Geometry: final body of the model. Coordinates: model frame, mm. A direction names the side the tool comes from. Round coordinates to 2 decimals unless told otherwise and drop trailing zeros. Loops run counter-clockwise (first coordinate to the right, second up) from the corner with the lowest first, then second, coordinate; pieces in that order, holes last. Notation, with made-up numbers: (-22, 77.5) - (27, 77.5) arc R31 ccw to (27, 106.5) - close; hole circle Ø3 at (8.5, 26.5). An arc over 180 degrees is marked (long way). Use CSV: the item, a comma, the result in double quotes.
Autodesk Inventor part; units mm, degrees
ref_plane "РабПлоскость4" through (-4.5219, -7.4249, -3) normal (0, 0, 1) x (1, 0, 0)
ref_plane "РабПлоскость5" through (-4.5219, -7.4249, -3) normal (0, 0, 1) x (1, 0, 0)
ref_plane "YZ Plane" through (0, 0, 0) normal (1, 0, 0) x (0, 1, 0)
sketch "Эскиз1" plane through (0, 0, 0) normal (0, 0, 1) x (1, 0, 0)
  arc A0 (0.3914, -1.6228) -> (0.394, 1.6268) centre (2.903, 0) ccw construction
  circle A1 centre (2.903, 0) radius 2.9903
  circle A2 centre (2.903, 0) radius 6
  point P0 (0, 0)
  dimension "d0" = 12
extrude "Выдавливание1" add sketch "Эскиз1" along normal blind 24
ref_plane "РабПлоскость2" through (3.6207, 5.9569, 0) normal (-0.1196, -0.9928, 0) x (0.9928, -0.1196, 0)
ref_plane "РабПлоскость1" through (5.8216, 7.5048, 10) normal (-0.1196, -0.9928, 0) x (0.9928, -0.1196, 0)
sketch "Эскиз2" plane through (3.6207, 5.9569, 0) normal (-0.1196, -0.9928, 0) x (0.9928, -0.1196, 0)
  line L0 (6, 0) -> (-6, 0)
  line L1 (0, 0) -> (0, 19.3984) construction
  line L2 (0, 12.5) -> (0, 16.5) construction
  line L3 (2, 12.5) -> (2, 16.5)
  line L4 (-2, 16.5) -> (-2, 12.5)
  arc A0 (-2, 12.5) -> (2, 12.5) centre (0, 12.5) ccw
  arc A1 (2, 16.5) -> (-2, 16.5) centre (0, 16.5) ccw
  point P0 (-2.8822, 0)
  point P1 (0, 14.5)
  dimension "d0" = 12
  dimension "d3" = 4
  dimension "d4" = 4
  dimension "d5" = 14.5
extrude "Выдавливание2" cut sketch "Эскиз2" along normal blind 2.5
ref_plane "РабПлоскость3" through (2.903, 0, 19) normal (0, 0, -1) x (-1, 0, 0)
sketch "Эскиз3" plane through (2.903, 0, 19) normal (0, 0, -1) x (-1, 0, 0)
  point P0 (2.903, 0)
sketch "Эскиз4" plane through (2.903, 0, 19) normal (0, 0, -1) x (-1, 0, 0)
  circle A0 centre (0, 0) radius 6.5
  point P0 (2.903, 0)
  dimension "d12" = 13
extrude "Выдавливание3" add sketch "Эскиз4" against normal blind 20
sketch "Эскиз5" plane through (2.903, 0, 39) normal (0, 0, 1) x (1, 0, 0)
  circle A0 centre (0, 0) radius 5
  circle A1 centre (0, 0) radius 7.2744
  point P0 (-2.903, 0)
  dimension "d15" = 10
extrude "Выдавливание4" cut sketch "Эскиз5" against normal blind 19
sketch "Эскиз6" plane through (2.903, 0, 0) normal (0, 0, -1) x (-1, 0, 0)
  circle A0 centre (0, 0) radius 3
  circle A1 centre (0, 0) radius 5
  point P0 (2.903, 0)
  dimension "d18" = 6
  dimension "d19" = 10
ref_plane "РабПлоскость4" through (-4.5219, -7.4249, -3) normal (0, 0, 1) x (1, 0, 0)
sketch "Эскиз8" plane through (2.903, 0, 0) normal (0, 0, -1) x (-1, 0, 0)
  circle A0 centre (0, 0) radius 6
  point P0 (2.903, 0)
extrude "Выдавливание6" cut sketch "Эскиз8" against normal blind 9
sketch "Эскиз9" plane through (2.903, 0, 9) normal (0, 0, -1) x (-1, 0, 0)
  circle A0 centre (0, 0) radius 3
  circle A1 centre (0, 0) radius 5
  point P0 (2.903, 0)
  dimension "d24" = 6
  dimension "d25" = 10
ref_plane "РабПлоскость5" through (-4.5219, -7.4249, -3) normal (0, 0, 1) x (1, 0, 0)
extrude "Выдавливание7" add sketch "Эскиз9" along normal up to surface (12 mm away)
sketch "Эскиз10" plane through (2.903, 0, 39) normal (0, 0, 1) x (1, 0, 0)
  circle A0 centre (0, 0) radius 5
  point P0 (-2.903, 0)
extrude "Выдавливание8" add sketch "Эскиз10" along normal blind 62
sketch "Эскиз11" plane through (2.903, 0, 101) normal (0, 0, 1) x (1, 0, 0)
  line L0 (3.5, 4.5942) -> (9.6944, 4.5942)
  line L1 (9.6944, 4.5942) -> (9.6944, -5.4033)
  line L2 (9.6944, -5.4033) -> (3.5, -5.4033)
  line L3 (3.5, -5.4033) -> (3.5, 4.5942)
  circle A0 centre (0, 0) radius 5
  point P0 (-2.903, 0)
  point P1 (3.5, 3.5707)
  point P2 (3.5, -3.5707)
  dimension "d30" = 3.5
extrude "Выдавливание9" cut sketch "Эскиз11" against normal blind 30 contours A0 L3 picked at (3.7121, 0.9363)
sketch "Эскиз12" plane through (2.903, 0, 20) normal (0, 0, 1) x (1, 0, 0)
  circle A0 centre (0, 0) radius 5.5
  point P0 (-2.903, 0)
  dimension "d33" = 11
extrude "Выдавливание10" add sketch "Эскиз12" along normal blind 38.8
sketch "Эскиз13" plane through (6.403, -3.5707, 101) normal (1, 0, 0) x (0, 0, -1)
  point P0 (101, 3.5707)
sketch "Эскиз14" plane through (6.403, -3.5707, 101) normal (1, 0, 0) x (0, 0, -1)
  point P0 (101, 3.5707)
sketch "Эскиз15" plane through (6.403, -3.5707, 101) normal (1, 0, 0) x (0, 0, -1)
  line L0 (30, 0) -> (30, 7.1414)
  line L1 (30, 3.5707) -> (0, 3.5707) construction
  line L2 (0, 8.5707) -> (0, -1.4293)
  point P0 (101, 3.5707)
  point P1 (0, 7.1414)
  point P2 (0, 0)
  point P3 (7, 3.5707)
  point P4 (23, 3.5707)
  dimension "d36" = 7
  dimension "d37" = 7
hole "Отверстие1" at (6.403, 0, 94) at (6.403, 0, 78) direction (-1, 0, 0) diameter 3.242 depth 11.8 tip angle 118
sketch "Эскиз16" plane through (2.903, 0, 9) normal (0, 0, -1) x (-1, 0, 0)
  circle A0 centre (0, 0) radius 6
  point P0 (2.903, 0)
extrude "Выдавливание11" add sketch "Эскиз16" along normal blind 1
ref_plane "РабПлоскость6" through (2.903, 0, 10) normal (0, 0, -1) x (0.9928, -0.1196, 0)
sketch "Эскиз17" plane through (2.903, 0, 10) normal (0, 0, -1) x (0.9928, -0.1196, 0)
  circle A0 centre (0, 0) radius 5.65
  circle A1 centre (0, 0) radius 7.5447
  point P0 (-2.8822, 0.3472)
  dimension "d47" = 11.3
extrude "Выдавливание12" cut sketch "Эскиз17" along normal blind 1.2
sketch "Эскиз18" plane through (0, 0, 0) normal (0, 1, 0) x (-1, 0, 0)
  line L0 (-7.903, -3) -> (2.097, -3) construction
  line L1 (2.097, -3) -> (-7.903, -3)
  line L2 (-2.903, -3) -> (-2.903, 1.2) construction
  point P0 (0, 0)
  dimension "d50" = 4.2
hole "Отверстие2" at (2.903, 0, 1.2) direction (0, 1, 0) diameter 2.459 depth 8.8 tip angle 118
properties part number "Вал вертикальной оси"
Item 1: Pin query (flat end, axial travel): P1, Ø6, axis at x = 4.5, y = 1, coming from the -Z side; P2, Ø5, axis at x = -0.5, z = 29.5, coming from the +Y side; P3, Ø2, axis at y = -5, z = 74.5, coming from the -X side; P4, Ø2, axis at y = 1, z = 81.5, coming from the +X side. Return the tip coordinate at first contact, or that it passes through.
Final values:
P1,"stops at z = -3"
P2,"stops at y = 5.43"
P3,"stops at x = -0.1"
P4,"stops at x = 6.4"
Item 2: Material intervals for line 1 (Z direction, x = 1.75, y = 0); line 2 (X direction, y = 4.05, z = 1.2); line 3 (Z direction, x = 2, y = 3.75), sorted ascending.
Final values:
line 1,"z = 8 to 9, 19 to 76.38, 79.62 to 92.38, 95.62 to 101"
line 2,"x = -0.03 to 1.67, 4.13 to 5.84"
line 3,"z = -3 to 0.37, 2.03 to 11.02, 17.98 to 101"
Item 3: Mould query, pull axis Y, two halves, no side actions, for faces 4 (the flat face through (5.438, 4.32, 14.472)), 5 (the flat face through (2, 0, 101)), 6 (the flat face through (3, 0, 8)). Classes: released by +Y, released by -Y, zero draft, split by the parting line, or undercut.
Final values:
face 4,"released by +Y"
face 5,"zero draft"
face 6,"undercut"
Item 4: Reachability of faces 1 (the cylindrical face through (-1.065, 3.042, 79.605)), 2 (the cylindrical face through (-0.775, 4.289, 9.408)), 3 (the cylindrical face through (2.12, -5.95, 14.44)) from +Z, -Z, +X, -X, +Y, -Y: full face, straight path, thin tool, end or side. Return the list, or none.
Final values:
face 1,"+Z"
face 2,"none"
face 3,"-Z"
Item 5: Section C-C on z = 1.2. Return the cut outline in (x, y), plus the area to 3 significant figures.
Final values:
outline,"(1.67, 2.74) - (1.67, 4.85) arc R5 ccw (long way) to (4.13, 4.85) - (4.13, 2.74) arc R3 cw (long way) to start"
area,"45.3 mm²"
Item 6: Section A-A on z = 34. Return the cut outline in (x, y).
Final values:
outline,"circle Ø11 at (2.9, 0)"
Item 7: Section B-B on z = 94. Return the cut outline in (x, y).
Final values:
outline,"(-1.83, -1.62) arc R5 ccw to (6.4, -3.57) - (6.4, -1.62) - close; (-1.83, 1.62) - (6.4, 1.62) - (6.4, 3.57) arc R5 ccw to start"
